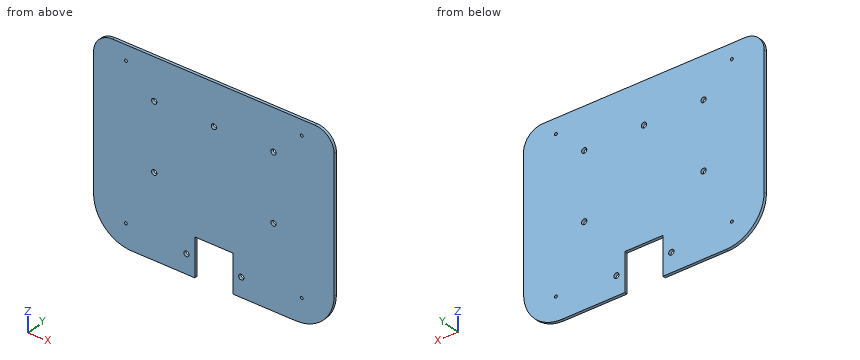
Autodesk Inventor part; units mm, degrees
ref_plane "YZ Plane" through (0, 0, 0) normal (1, 0, 0) x (0, 1, 0)
ref_plane "XZ Plane" through (0, 0, 0) normal (0, 1, 0) x (-1, 0, 0)
ref_plane "XY Plane" through (0, 0, 0) normal (0, 0, 1) x (1, 0, 0)
sketch "Sketch1" plane through (0, 0, 0) normal (0, 1, 0) x (-1, 0, 0)
  line L0 (126, -23.5) -> (126, 23.5)
  line L1 (126, 23.5) -> (-126, 23.5)
  line L2 (-126, 23.5) -> (-126, -23.5)
  line L3 (82.5, -115.5) -> (82.5, -33.5)
  line L4 (0, 23.5) -> (0, -23.5) construction
  line L5 (-82.5, -115.5) -> (-82.5, -33.5)
  line L6 (42.5, -155.5) -> (-42.5, -155.5)
  line L7 (-126, -23.5) -> (-92.5, -23.5)
  line L8 (92.5, -23.5) -> (126, -23.5)
  arc A0 (-82.5, -33.5) -> (-92.5, -23.5) centre (-92.5, -33.5) ccw
  arc A1 (92.5, -23.5) -> (82.5, -33.5) centre (92.5, -33.5) ccw
  line L9 (0, 23.5) -> (0, -155.5) construction
  line L10 (20, -155.5) -> (-20, -155.5)
  line L11 (-20, -155.5) -> (-20, -115.5)
  line L12 (-20, -115.5) -> (20, -115.5)
  line L13 (20, -115.5) -> (20, -155.5)
  circle A2 centre (0, 0) radius 2.75
  circle A3 centre (62.5, 0) radius 2.75
  circle A4 centre (-62.5, 0) radius 2.75
  circle A5 centre (62.5, -69.5) radius 2.75
  circle A6 centre (-62.5, -69.5) radius 2.75
  circle A7 centre (28.75, -135.5) radius 2.75
  circle A8 centre (-28.75, -135.5) radius 2.75
  line L14 (82.5, -115.5) -> (82.5, -155.5)
  line L15 (82.5, -155.5) -> (42.5, -155.5)
  line L16 (-42.5, -155.5) -> (-82.5, -155.5)
  line L17 (-82.5, -155.5) -> (-82.5, -115.5)
  line L18 (126, -23.5) -> (-126, -23.5)
  line L19 (-126, -23.5) -> (-126, -155.5)
  line L20 (-126, -155.5) -> (126, -155.5)
  line L21 (126, -155.5) -> (126, -23.5)
  line L22 (126, 23.5) -> (-126, 23.5)
  line L23 (-126, 23.5) -> (-126, 43.5)
  line L24 (-126, 43.5) -> (126, 43.5)
  line L25 (126, 43.5) -> (126, 23.5)
  point P0 (82.5, -23.5)
  point P1 (-82.5, -23.5)
  point P2 (0, -135.5)
  dimension "d0" = 252
  dimension "d1" = 47
  dimension "d4" = 10
  dimension "d5" = 40
  dimension "d6" = 40
  dimension "d7" = 5.5
  dimension "d8" = 5.5
  dimension "d9" = 5.5
  dimension "d10" = 5.5
  dimension "d16" = 20
extrude "Extrusion1" add sketch "Sketch1" along normal blind 3 contours L8 L18 L7 L2 L1 L0 | L21 L20 L14 L3 A1 L8 | L1 L23 L24 L25 | A1 L3 L14 L15 L6 L13 L12 L11 L16 L17 L5 A0 L18 | A0 L5 L17 L20 L19 L7
fillet "Fillet3" radius 40 2 edges at (126, 1.5, -155.5) (-126, 1.5, -155.5)
fillet "Fillet4" radius 20 2 edges at (126, 1.5, 43.5) (-126, 1.5, 43.5)
sketch "Sketch2" plane through (0, 3, 0) normal (0, 1, 0) x (1, 0, 0)
  line L0 (-92.17, 130.7671) -> (92.17, 130.7671) construction
  line L1 (92.17, 130.7671) -> (92.17, -27.8329) construction
  line L2 (92.17, -27.8329) -> (-92.17, -27.8329) construction
  line L3 (-92.17, -27.8329) -> (-92.17, 130.7671) construction
  line L4 (0, 150.8633) -> (0, -88.711) construction
  line L5 (20, 115.5) -> (-20, 115.5)
  circle A0 centre (-92.17, 130.7671) radius 1.5
  circle A1 centre (92.17, 130.7671) radius 1.5
  circle A2 centre (-92.17, -27.8329) radius 1.5
  circle A3 centre (92.17, -27.8329) radius 1.5
  point P0 (0, 0)
  point P1 (0, 115.5)
  dimension "d18" = 184.34
  dimension "d19" = 158.6
  dimension "d20" = 3
extrude "Extrusion2" cut sketch "Sketch2" against normal through all
equation "\"d21\" = d19"
properties part number "Chassis Rear Plate"
Geometry: final body of the model. Coordinates: model frame, mm. Round coordinates to 2 decimals unless told otherwise and drop trailing zeros. Order: outer loops, then holes, each group sorted by start corner. A loop starts at its lowest first (then second) coordinate and runs counter-clockwise, first axis right, second up. Notation, with made-up numbers: (-33.5, -38) -> (-19.5, -38) arc R14 ccw to (-19.5, -19) -> close; hole circle Ø2 at (-1, -4). An arc over 180 degrees is marked (long way). Put each result on its own line as item: value. Start each with the question number.
Q1. Section B-B on x = 28.75. Return the cut outline in (y, z).
Q2. Section C-C on x = -62.5. Return the cut outline in (y, z).
Q3. Section A-A on z = 0. Return the cut outline in (x, y).
Q4. Line query: probe 1 along Z at (x, y) = (-62.5, 1.95); probe 2 along Z at (x, y) = (-28.75, 1.1); probe 3 along X at (y, z) = (2.15, -135.5). Output: solid intervals per line, ascending.
Q5. First-contact query: pin 1 (2 mm diameter, centred on x = 6.5, z = -49, fed in from -Y); pin 2 (1.5 mm diameter, centred on y = 1, z = -129, fed in from -X); pin 3 (1.5 mm diameter, centred on x = -6, y = 1, fed in from -Z). Flat tips, straight axial feed; report the tip coordinate or a pass-through.
Q6. Section D-D on z = -69.5. Return the cut outline in (x, y).
Ans:
1. outline: (0, -155.5) -> (3, -155.5) -> (3, -138.25) -> (0, -138.25) -> close; (0, -132.75) -> (3, -132.75) -> (3, 43.5) -> (0, 43.5) -> close
2. outline: (0, -155.5) -> (3, -155.5) -> (3, -72.25) -> (0, -72.25) -> close; (0, -66.75) -> (3, -66.75) -> (3, -2.75) -> (0, -2.75) -> close; (0, 2.75) -> (3, 2.75) -> (3, 43.5) -> (0, 43.5) -> close
3. outline: (-126, 0) -> (-65.25, 0) -> (-65.25, 3) -> (-126, 3) -> close; (-59.75, 0) -> (-2.75, 0) -> (-2.75, 3) -> (-59.75, 3) -> close; (2.75, 0) -> (59.75, 0) -> (59.75, 3) -> (2.75, 3) -> close; (65.25, 0) -> (126, 0) -> (126, 3) -> (65.25, 3) -> close
4. probe 1: z = -155.5 to -72.25, -66.75 to -2.75, 2.75 to 43.5
4. probe 2: z = -155.5 to -138.25, -132.75 to 43.5
4. probe 3: x = -120.64 to -31.5, -26 to -20, 20 to 26, 31.5 to 120.64
5. pin 1: stops at y = 0
5. pin 2: stops at x = -123.91
5. pin 3: stops at z = -115.5
6. outline: (-126, 0) -> (-65.25, 0) -> (-65.25, 3) -> (-126, 3) -> close; (-59.75, 0) -> (59.75, 0) -> (59.75, 3) -> (-59.75, 3) -> close; (65.25, 0) -> (126, 0) -> (126, 3) -> (65.25, 3) -> close
